Source: CAD feature listing. Evaluate the final solid. Frame: model axes, mm. A direction names the side the tool comes from. Coordinates: 2 decimals unless noted, no trailing zeros. Order: outer loops, then holes, each group sorted by start corner. A loop starts at its lowest first (then second) coordinate and runs counter-clockwise, first axis right, second up.
Autodesk Fusion 360 part; units mm, degrees
sketch "Sketch1" plane through (0, 0, 0) normal (0, 0, 1) x (1, 0, 0)
  line L0 (0, 0) -> (300, 0)
  line L1 (300, 0) -> (300, 260)
  line L2 (300, 260) -> (0, 260)
  line L3 (0, 260) -> (0, 0)
  line L4 (5, 5) -> (295, 5)
  line L5 (295, 5) -> (295, 255)
  line L6 (295, 255) -> (5, 255)
  line L7 (5, 255) -> (5, 5)
  circle A0 centre (7.5, 22.5) radius 2.5
  circle A1 centre (7.5, 237.5) radius 2.5
  circle A2 centre (292.5, 237.5) radius 2.5
  circle A3 centre (292.5, 22.5) radius 2.5
  circle A4 centre (7.5, 237.5) radius 6.5
  circle A5 centre (292.5, 237.5) radius 6.5
  circle A6 centre (292.5, 22.5) radius 6.5
  circle A7 centre (7.5, 22.5) radius 6.5
  dimension "d1" = 300
  dimension "d2" = 260
  dimension "d3" = 290
  dimension "d4" = 250
  dimension "d5" = 5
  dimension "d6" = 5
  dimension "d7" = 5
  dimension "d8" = 5
  dimension "d9" = 5
  dimension "d10" = 5
  dimension "d11" = 5
  dimension "d12" = 5
  dimension "d13" = 22.5
  dimension "d16" = 22.5
  dimension "d17" = 7.5
  dimension "d18" = 7.5
  dimension "d19" = 7.5
  dimension "d20" = 22.5
  dimension "d21" = 7.5
  dimension "d22" = 22.5
  dimension "d23" = 13
  dimension "d24" = 7.5
  dimension "d25" = 22.5
  dimension "d26" = 13
  dimension "d27" = 7.5
  dimension "d28" = 22.5
  dimension "d29" = 13
  dimension "d30" = 7.5
  dimension "d31" = 22.5
  dimension "d32" = 13
  dimension "d33" = 7.5
  dimension "d34" = 22.5
extrude "Extrude1" add sketch "Sketch1" along normal blind 80 contours L7 A7 picked at (9.3974, 27.2942) makes body 1
extrude "Extrude2" add sketch "Sketch1" along normal blind 80 separate body contours L5 A6 picked at (287.3448, 22.5) makes body 2
extrude "Extrude3" add sketch "Sketch1" along normal blind 80 separate body contours L5 A5 picked at (287.3448, 237.5) makes body 3
extrude "Extrude4" add sketch "Sketch1" along normal blind 80 separate body contours L7 A4 picked at (9.3974, 242.2942) makes body 4
extrude "Extrude5" add sketch "Sketch1" along normal blind 80 separate body contours L0 L1 L2 L3 makes body 5
extrude "Extrude6" add sketch "Sketch1" along normal blind 80 contours L7 A4 picked at (2.3567, 237.1826) bodies 4 5
extrude "Extrude7" add sketch "Sketch1" along normal blind 80 contours L7 A7 picked at (2.3567, 22.1826) bodies 1 4
extrude "Extrude8" add sketch "Sketch1" along normal blind 80 contours L5 A6 picked at (297.6433, 22.8174) bodies 1 2
extrude "Extrude9" add sketch "Sketch1" along normal blind 80 contours L5 A5 picked at (297.6433, 237.1826) bodies 1 3
sketch "Sketch2" plane through (5, 0, 0) normal (1, 0, 0) x (0, 1, 0)
  line L0 (28.5, 0) -> (231.5, 0)
  line L1 (231.5, 0) -> (231.5, 80)
  line L2 (231.5, 80) -> (28.5, 80)
  line L3 (28.5, 80) -> (28.5, 0)
  line L4 (35, 30) -> (89.718, 30)
  line L5 (89.718, 30) -> (89.718, 0)
  line L6 (89.718, 0) -> (35, 0)
  line L7 (35, 0) -> (35, 30)
  line L8 (5, 0) -> (5, 80)
  line L9 (67.238, 17.75) -> (79.758, 17.75)
  line L10 (79.758, 17.75) -> (79.758, 6.39)
  line L11 (79.758, 6.39) -> (67.238, 6.39)
  line L12 (67.238, 6.39) -> (67.238, 17.75)
  line L13 (38.153, 17.75) -> (48.153, 17.75)
  line L14 (48.153, 17.75) -> (48.153, 6.15)
  line L15 (48.153, 6.15) -> (38.153, 6.15)
  line L16 (38.153, 6.15) -> (38.153, 17.75)
  dimension "d53" = 54.718
  dimension "d56" = 30
  dimension "d57" = 50
  dimension "d58" = 30
  dimension "d59" = 12.52
  dimension "d60" = 10
  dimension "d61" = 9.96
  dimension "d62" = 6.39
  dimension "d63" = 6.15
  dimension "d64" = 19.085
  dimension "d65" = 11.36
  dimension "d66" = 11.6
extrude "Extrude10" cut sketch "Sketch2" against normal blind 5 contours L9 L10 L11 L12 bodies 1
extrude "Extrude11" cut sketch "Sketch2" against normal blind 5 contours L13 L14 L15 L16 bodies 1
sketch "Sketch3" plane through (0, 260, 0) normal (0, 1, 0) x (-1, 0, 0)
  line L0 (-300, 0) -> (0, 0)
  line L1 (0, 0) -> (0, 80)
  line L2 (0, 80) -> (-300, 80)
  line L3 (-300, 80) -> (-300, 0)
  line L4 (-295, 80) -> (-5, 80)
  line L5 (-5, 80) -> (-5, 40)
  line L6 (-5, 40) -> (-295, 40)
  line L7 (-295, 40) -> (-295, 80)
  line L8 (-300, 0) -> (0, 0)
  line L9 (-295, 40) -> (-300, 40)
  line L10 (-300, 40) -> (-300, 80)
  line L11 (-300, 80) -> (-295, 80)
  line L12 (-295, 80) -> (-295, 40)
  line L13 (-5, 40) -> (0, 40)
  line L14 (0, 40) -> (0, 80)
  line L15 (0, 80) -> (-5, 80)
  line L16 (-5, 80) -> (-5, 40)
  dimension "d71" = 290
  dimension "d72" = 5
  dimension "d73" = 5
  dimension "d74" = 40
  dimension "d92" = 5
  dimension "d93" = 40
  dimension "d94" = 5
  dimension "d95" = 40
extrude "Extrude12" cut sketch "Sketch3" against normal blind 5 contours L2 L4 L5 L6 L7 L12 L16 bodies 1
sketch "Sketch4" plane through (0, 0, 0) normal (0, -1, 0) x (1, 0, 0)
  line L0 (0, 0) -> (300, 0)
  line L1 (300, 0) -> (300, 80)
  line L2 (300, 80) -> (0, 80)
  line L3 (0, 80) -> (0, 0)
  line L4 (5, 80) -> (295, 80)
  line L5 (295, 80) -> (295, 40)
  line L6 (295, 40) -> (5, 40)
  line L7 (5, 40) -> (5, 80)
  line L8 (0, 0) -> (300, 0)
  line L9 (5, 80) -> (0, 80)
  line L10 (0, 80) -> (0, 40)
  line L11 (0, 40) -> (5, 40)
  line L12 (5, 40) -> (5, 80)
  line L13 (295, 40) -> (300, 40)
  line L14 (300, 40) -> (300, 80)
  line L15 (300, 80) -> (295, 80)
  line L16 (295, 80) -> (295, 40)
  dimension "d77" = 290
  dimension "d78" = 40
  dimension "d79" = 40
  dimension "d80" = 5
  dimension "d81" = 5
  dimension "d84" = 5
  dimension "d85" = 40
  dimension "d86" = 5
  dimension "d87" = 40
extrude "Extrude13" cut sketch "Sketch4" against normal blind 5 contours L2 L4 L5 L6 L7 L12 L16 bodies 1
sketch "Sketch5" plane through (0, 0, 0) normal (-1, 0, 0) x (0, -1, 0)
  line L0 (-48.153, 6.15) -> (-48.153, 17.75)
  line L1 (-48.153, 17.75) -> (-38.153, 17.75)
  line L2 (-38.153, 17.75) -> (-38.153, 6.15)
  line L3 (-38.153, 6.15) -> (-48.153, 6.15)
  line L4 (-79.758, 6.39) -> (-79.758, 17.75)
  line L5 (-79.758, 17.75) -> (-67.238, 17.75)
  line L6 (-67.238, 17.75) -> (-67.238, 6.39)
  line L7 (-67.238, 6.39) -> (-79.758, 6.39)
  line L8 (-260, 0) -> (0, 0)
  line L9 (0, 0) -> (0, 80)
  line L10 (0, 80) -> (-260, 80)
  line L11 (-260, 80) -> (-260, 0)
extrude "Extrude14" cut sketch "Sketch4" against normal blind 5 contours L1 L2 L5 L13 L14 L15 L16 bodies 1
extrude "Extrude15" cut sketch "Sketch4" against normal blind 5 contours L2 L3 L7 L9 L10 L11 L12 bodies 1
extrude "Extrude16" cut sketch "Sketch3" against normal blind 5 contours L1 L2 L5 L13 L14 L15 L16 bodies 1
extrude "Extrude17" cut sketch "Sketch3" against normal blind 5 contours L2 L3 L7 L9 L10 L11 L12 bodies 1
fillet "Fillet1" radius 15 1 edges at (297.5, 5, 80) on bodies 1
fillet "Fillet2" radius 15 1 edges at (297.5, 255, 80) on bodies 1
fillet "Fillet3" radius 15 1 edges at (2.5, 255, 80) on bodies 1
fillet "Fillet4" radius 15 1 edges at (2.5, 5, 80) on bodies 1
1. Section query A-A on y = 148.5. Return loops of the section in (x, z), plus the area to 3 significant figures.
Findings:
outline: (0, 0) - (5, 0) - (5, 80) - (0, 80) - close; (295, 0) - (300, 0) - (300, 80) - (295, 80) - close
area: 800 mm2
2. Section query C-C on x = 86.5. Return loops of the section in (y, z).
Findings:
outline: (0, 0) - (5, 0) - (5, 40) - (0, 40) - close; (255, 0) - (260, 0) - (260, 40) - (255, 40) - close
3. Access query for faces 1 (the face through (4, 11, 77)), 2 (the face through (295, 11, 39)). Directions: +Z, -Z, +X, -X, +Y, -Y. A direction counts if a zero-diameter tool reaches every point of the face in a straight line with its end or side. Return the directions, or none.
Findings:
face 1: +Z, +X, -X, -Y
face 2: +Z, -Z
4. Section query B-B on z = 70.5. Return loops of the section in (x, y), plus the area to 3 significant figures.
Findings:
outline: (0, 6.04) - (5, 6.04) - (5, 16.5) arc R6.5 ccw (long way) to (5, 28.5) - (5, 231.5) arc R6.5 ccw (long way) to (5, 243.5) - (5, 253.96) - (0, 253.96) - close; (295, 6.04) - (300, 6.04) - (300, 253.96) - (295, 253.96) - (295, 243.5) arc R6.5 ccw (long way) to (295, 231.5) - (295, 28.5) arc R6.5 ccw (long way) to (295, 16.5) - close; hole circle Ø5 at (7.5, 22.5); hole circle Ø5 at (7.5, 237.5); hole circle Ø5 at (292.5, 22.5); hole circle Ø5 at (292.5, 237.5)
area: 2,790 mm2
5. Section query D-D on z = 31. Return loops of the section in (x, y).
Findings:
outline: (0, 0) - (300, 0) - (300, 260) - (0, 260) - close; hole (5, 5) - (295, 5) - (295, 16.5) arc R6.5 cw (long way) to (295, 28.5) - (295, 231.5) arc R6.5 cw (long way) to (295, 243.5) - (295, 255) - (5, 255) - (5, 243.5) arc R6.5 cw (long way) to (5, 231.5) - (5, 28.5) arc R6.5 cw (long way) to (5, 16.5) - close; hole circle Ø5 at (7.5, 22.5); hole circle Ø5 at (7.5, 237.5); hole circle Ø5 at (292.5, 22.5); hole circle Ø5 at (292.5, 237.5)
6. Pin query (flat end, axial travel): P1, Ø1.5, axis at x = 3, y = 72.5, coming from the -Z side; P2, Ø4, axis at x = 152.5, y = 1.5, coming from the +Z side; P3, Ø4.5, axis at x = 292.5, y = 237.5, coming from the +Z side; P4, Ø2.5, axis at x = 2, z = 50, coming from the -Y side. Return the tip coordinate at first contact, or that it passes through.
Findings:
P1: stops at z = 0
P2: stops at z = 40
P3: passes through
P4: stops at y = 5
7. Ray query, line 1 (X direction, y = 22.5, z = 59.5); line 2 (X direction, y = 22, z = 32); line 3 (Y direction, x = 292, z = 61). Return the intervals inside material, ascending.
Findings:
line 1: x = 0 to 5, 10 to 14, 286 to 290, 295 to 300
line 2: x = 0 to 5.05, 9.95 to 13.98, 286.02 to 290.05, 294.95 to 300
line 3: y = 16.02 to 20.05, 24.95 to 28.98, 231.02 to 235.05, 239.95 to 243.98
